from build123d import *

# Parameters (mm, degrees)
F0_W     = 100
F0_H     = 50
F1_DEPTH = 40
F2_R     = 15
F3_DEPTH = 10
F4_R     = 15
F5_DEPTH = 30


with BuildPart() as f1:
    # F0 (on Front) → F1 (new body)
    with BuildSketch(Plane.XZ):
        Rectangle(F0_W, F0_H)
    extrude(amount=F1_DEPTH)

    # F2 (on face) → F3 (join)
    with BuildSketch(Plane.XY.offset(25)):
        with Locations((-32.5, -20)):
            Circle(F2_R)
        with Locations((32.5, -20)):
            Circle(F2_R)
    extrude(amount=F3_DEPTH)

    # F4 (on face) → F5 (cut)
    with BuildSketch(Plane(origin=(0, 0, -25), x_dir=(1, 0, 0), z_dir=(0, 0, -1))):
        with Locations((-32.5, 20)):
            Circle(F4_R)
        with Locations((32.5, 20)):
            Circle(F4_R)
    extrude(amount=-F5_DEPTH, mode=Mode.SUBTRACT)


solid = f1.part
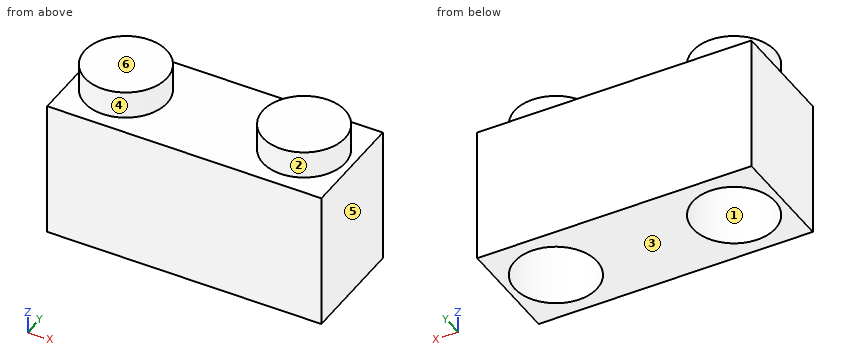
Could you check a few things on this model? Use its own coordinates, in mm. Face numbers are marked on the shaded views. A direction names the side the tool comes from. Round coordinates to 2 decimals unless told otherwise and drop trailing zeros. Order: outer loops, then holes, each group sorted by start corner. A loop starts at its lowest first (then second) coordinate and runs counter-clockwise, first axis right, second up. Notation, with made-up numbers: M -29.75,30 L -0.75,30 A33 ccw -0.75,68 Z; hole C 77,60.25 d9. An arc over 180 degrees is marked long. One line per item, written item: value.
(1) I'm going to push a flat-ended pin straight in: P1, Ø3, axis at x = 35, y = -15.5, coming from the -Z side. Where does the tip first touch, or does it pass through?
Ans:
P1: stops at z = 5
(2) Imagine slicing it at C-C (y = -20). Write out the boundary of the cut face in (x, z).
Ans:
outline: M -50,-25 L -47.5,-25 L -47.5,5 L -17.5,5 L -17.5,-25 L 17.5,-25 L 17.5,5 L 47.5,5 L 47.5,-25 L 50,-25 L 50,25 L 47.5,25 L 47.5,35 L 17.5,35 L 17.5,25 L -17.5,25 L -17.5,35 L -47.5,35 L -47.5,25 L -50,25 Z
(3) Imagine slicing it at D-D (z = 28.5). Write out the boundary of the cut face in (x, y).
Ans:
outline: C -32.5,-20 d30; C 32.5,-20 d30
(4) Imagine slicing it at B-B (x = 32.5). Write out the boundary of the cut face in (y, z).
Ans:
outline: M -40,-25 L -35,-25 L -35,5 L -5,5 L -5,-25 L 0,-25 L 0,25 L -5,25 L -5,35 L -35,35 L -35,25 L -40,25 Z
(5) If we mould it in two halves opening along X, with no side actions, what happens to the marked faces 4, 5 and 6? For each: released by +X, released by -X, zero draft, split by the parting line, or undercut.
Ans:
face 4: undercut
face 5: released by +X
face 6: zero draft
(6) Imagine slicing it at A-A (z = -17). Write out the boundary of the cut face in (x, y), and give its area (3 significant figures).
Ans:
outline: M -50,-40 L 50,-40 L 50,0 L -50,0 Z; hole C -32.5,-20 d30; hole C 32.5,-20 d30
area: 2,590 mm^2
(7) I need wall thicknesses on line 1 along X through (y, z) = (-20, -17.5); line 2 along X through (y, z) = (-24.5, -4.5); line 3 along Y through (x, z) = (-32.5, -7.5). Which ranges of each line are inside material? Lowest first, please. Write a range as from..to.
Ans:
line 1: x = -50..-47.5, -17.5..17.5, 47.5..50
line 2: x = -50..-46.81, -18.19..18.19, 46.81..50
line 3: y = -40..-35, -5..0
(8) Which directions (+Z, -Z, +X, -X, +Y, -Y) give clear straight access to the entire face, cutting with the end or side of a thin tool? Please do the marked faces 1, 2 and 3.
Ans:
face 1: -Z
face 2: +Z
face 3: -Z, +X, -X, +Y, -Y
